from build123d import *

# Parameters (mm, degrees)
SKETCH1_W                      = 370
SKETCH1_H                      = 370
BOSS_EXTRUDE1_DEPTH            = 6.35
CUT_EXTRUDE2_REACH             = 263.707
CUT_EXTRUDE2_DIRECTION_2_DEPTH = 262.706558


with BuildPart() as part:
    # Sketch1 → Boss-Extrude1 (new body)
    with BuildSketch(Plane(origin=(0, 0, 0), x_dir=(1, 0, 0), z_dir=(0, 1, 0))):
        Rectangle(SKETCH1_W, SKETCH1_H)
    extrude(amount=BOSS_EXTRUDE1_DEPTH)

    # Sketch2 → Cut-Extrude2 (cut, up to next)
    with BuildSketch(Plane(origin=(0, 0, 0), x_dir=(1, 0, 0), z_dir=(0, 1, 0)), mode=Mode.PRIVATE) as cut_extrude2_sk1:
        with BuildLine():
            Line((-185, 185), (-185, 160))
            Line((-185, 160), (-165, 160))
            ThreePointArc((-165, 160), (-161.464466094, 161.464466094), (-160, 165))
            Line((-160, 165), (-160, 185))
            Line((-160, 185), (-185, 185))
        make_face()
    cut_extrude2_tool1 = extrude(cut_extrude2_sk1.sketch, amount=CUT_EXTRUDE2_REACH, mode=Mode.PRIVATE) & part.part
    # Sketch2 → Cut-Extrude2 (cut, up to next)
    with BuildSketch(Plane(origin=(0, 0, 0), x_dir=(1, 0, 0), z_dir=(0, 1, 0)), mode=Mode.PRIVATE) as cut_extrude2_sk2:
        with BuildLine():
            Line((-185, -185), (-160, -185))
            Line((-160, -185), (-160, -165))
            ThreePointArc((-160, -165), (-161.464466094, -161.464466094), (-165, -160))
            Line((-165, -160), (-185, -160))
            Line((-185, -160), (-185, -185))
        make_face()
    cut_extrude2_tool2 = extrude(cut_extrude2_sk2.sketch, amount=CUT_EXTRUDE2_REACH, mode=Mode.PRIVATE) & part.part
    # Sketch2 → Cut-Extrude2 (cut, up to next)
    with BuildSketch(Plane(origin=(0, 0, 0), x_dir=(1, 0, 0), z_dir=(0, 1, 0)), mode=Mode.PRIVATE) as cut_extrude2_sk3:
        with BuildLine():
            Line((185, 185), (160, 185))
            Line((160, 185), (160, 165))
            ThreePointArc((160, 165), (161.464466094, 161.464466094), (165, 160))
            Line((165, 160), (185, 160))
            Line((185, 160), (185, 185))
        make_face()
    cut_extrude2_tool3 = extrude(cut_extrude2_sk3.sketch, amount=CUT_EXTRUDE2_REACH, mode=Mode.PRIVATE) & part.part
    # Sketch2 → Cut-Extrude2 (cut, up to next)
    with BuildSketch(Plane(origin=(0, 0, 0), x_dir=(1, 0, 0), z_dir=(0, 1, 0)), mode=Mode.PRIVATE) as cut_extrude2_sk4:
        with BuildLine():
            Line((185, -185), (185, -160))
            Line((185, -160), (165, -160))
            ThreePointArc((165, -160), (161.464466094, -161.464466094), (160, -165))
            Line((160, -165), (160, -185))
            Line((160, -185), (185, -185))
        make_face()
    cut_extrude2_tool4 = extrude(cut_extrude2_sk4.sketch, amount=CUT_EXTRUDE2_REACH, mode=Mode.PRIVATE) & part.part
    add(cut_extrude2_tool1.solids().sort_by_distance((-172.59856, 0, -172.59856))[0], mode=Mode.SUBTRACT)
    add(cut_extrude2_tool2.solids().sort_by_distance((-172.59856, 0, 172.59856))[0], mode=Mode.SUBTRACT)
    add(cut_extrude2_tool3.solids().sort_by_distance((172.59856, 0, -172.59856))[0], mode=Mode.SUBTRACT)
    add(cut_extrude2_tool4.solids().sort_by_distance((172.59856, 0, 172.59856))[0], mode=Mode.SUBTRACT)

    # Sketch2 → Cut-Extrude2 direction 2 (cut)
    with BuildSketch(Plane(origin=(0, 0, 0), x_dir=(1, 0, 0), z_dir=(0, 1, 0))):
        with BuildLine():
            Line((-185, 185), (-185, 160))
            Line((-185, 160), (-165, 160))
            ThreePointArc((-165, 160), (-161.464466094, 161.464466094), (-160, 165))
            Line((-160, 165), (-160, 185))
            Line((-160, 185), (-185, 185))
        make_face()
        with BuildLine():
            Line((-185, -185), (-160, -185))
            Line((-160, -185), (-160, -165))
            ThreePointArc((-160, -165), (-161.464466094, -161.464466094), (-165, -160))
            Line((-165, -160), (-185, -160))
            Line((-185, -160), (-185, -185))
        make_face()
        with BuildLine():
            Line((185, 185), (160, 185))
            Line((160, 185), (160, 165))
            ThreePointArc((160, 165), (161.464466094, 161.464466094), (165, 160))
            Line((165, 160), (185, 160))
            Line((185, 160), (185, 185))
        make_face()
        with BuildLine():
            Line((185, -185), (185, -160))
            Line((185, -160), (165, -160))
            ThreePointArc((165, -160), (161.464466094, -161.464466094), (160, -165))
            Line((160, -165), (160, -185))
            Line((160, -185), (185, -185))
        make_face()
    extrude(amount=-CUT_EXTRUDE2_DIRECTION_2_DEPTH, mode=Mode.SUBTRACT)


solid = part.part
Geometry check sheet. Reference: the model listing, model coordinates, mm. Give positions to 0.01 mm unless a question says otherwise; leave off trailing zeros. Order: outer loops, then holes, each group sorted by start corner. A loop starts at its lowest first (then second) coordinate and runs counter-clockwise, first axis right, second up.
1) Material ranges on probe 1 along Z at (x, y) = (170, 2.25), recorded low to high.
Results are:
probe 1: z = -160 to 160
2) Cross-section at A-A (y = 2.25). Record the boundary of the cut face in (x, z), then the cut area to 3 significant figures.
Results are:
outline: (-185, -160) - (-165, -160) arc R5 cw to (-160, -165) - (-160, -185) - (160, -185) - (160, -165) arc R5 cw to (165, -160) - (185, -160) - (185, 160) - (165, 160) arc R5 cw to (160, 165) - (160, 185) - (-160, 185) - (-160, 165) arc R5 cw to (-165, 160) - (-185, 160) - close
area: 134,000 mm2
3) Gauge pin test, flat ends, axial feed: pin 1 (3 mm diameter, centred on x = 175.5, y = 4, fed in from -Z); pin 2 (3 mm diameter, centred on y = 4, z = -170.5, fed in from -X); pin 3 (1.9 mm diameter, centred on y = 4.5, z = 172, fed in from +X). Record the tip position at first contact, or that the pin passes through.
Results are:
pin 1: stops at z = -160
pin 2: stops at x = -160
pin 3: stops at x = 160
